from build123d import *

# Parameters (mm, degrees)
F1_DEPTH = 28
F3_DEPTH = 244
F5_DEPTH = 28
F6_R     = 2
F7_R     = 1
F8_R     = 4.25
F9_DEPTH = 25


with BuildPart() as f1:
    # F0 (on Top) → F1 (new body)
    with BuildSketch(Plane.XY):
        Polygon((-19.75, -17.750001), (-19.75, -19.75), (-9.25, -19.75), (19.75, 9.25), (19.75, 19.75), (17.750001, 19.75), (17.750001, 10.078427), (-10.078427, -17.750001), align=None)
    extrude(amount=F1_DEPTH)

    # F2 (on face) → F3 (join)
    with BuildSketch(Plane.XY.offset(28)):
        Polygon((-19.75, -19.75), (-9.25, -19.75), (19.75, 9.25), (19.75, 19.75), (11.25, 19.75), (11.25, 24.25), (9.25, 26.25), (9.25, 23.421573), (9.25, 19.75), (9.25, 17.750001), (17.750001, 17.750001), (17.750001, 10.078427), (16.585787, 8.914213), (-8.914213, -16.585787), (-10.078427, -17.750001), (-17.750001, -17.750001), (-17.750001, -9.25), (-19.75, -9.25), (-23.421573, -9.25), (-26.25, -9.25), (-24.25, -11.25), (-19.75, -11.25), align=None)
    extrude(amount=F3_DEPTH)

    # F4 (on face) → F5 (join)
    with BuildSketch(Plane.XY.offset(272)):
        Polygon((19.75, 9.25), (19.75, 19.75), (17.750001, 19.75), (17.750001, 10.078427), (-10.078427, -17.750001), (-19.75, -17.750001), (-19.75, -19.75), (-9.25, -19.75), align=None)
    extrude(amount=F5_DEPTH)

    # F6
    f6_edges = [f1.edges().sort_by_distance(p)[0] for p in [
        (19.75, 9.25, 150),
        (-9.25, -19.75, 150),
    ]]
    fillet(f6_edges, radius=F6_R)

    # F7
    f7_edges = [f1.edges().sort_by_distance(p)[0] for p in [
        (-19.75, -19.75, 150),
        (19.75, 19.75, 150),
    ]]
    fillet(f7_edges, radius=F7_R)

    # F8 (on face) → F9 (cut)
    with BuildSketch(Plane(origin=(5.25, -5.25, 0), x_dir=(0.707107, 0.707107, 0), z_dir=(0.707107, -0.707107, 0))):
        with Locations((0, 286)):
            Circle(F8_R)
    extrude(amount=-F9_DEPTH, mode=Mode.SUBTRACT)


solid = f1.part
Geometry check sheet. Reference: the model listing, model coordinates, mm. A direction names the side the tool comes from. Coordinates: 2 decimals unless noted, no trailing zeros. Order: outer loops, then holes, each group sorted by start corner. A loop starts at its lowest first (then second) coordinate and runs counter-clockwise, first axis right, second up. Notation, with made-up numbers: (-9.75, 39.5) - (45.25, 39.5) arc R17 cw to (45.25, 46.5) - close; hole circle Ø10 at (-22, 81). An arc over 180 degrees is marked (long way). Answer in a Markdown table with one row per item. Add a question column.
1) Gauge pin test, flat ends, axial feed: P1, Ø10.5, axis at y = 16, z = 159, coming from the -X side; P2, Ø1.3, axis at x = -22, z = 137.5, coming from the -Y side; P3, Ø7, axis at y = -14, z = 188.5, coming from the +X side; P4, Ø8, axis at x = 13.5, y = 10, coming from the +Z side. Record the tip position at first contact, or that the pin passes through.
2) Material ranges on line 1 along X through (y, z) = (18, 220); line 2 along Y through (x, z) = (13.5, 67); line 3 along Y through (x, z) = (16.5, 79), recorded low to high. Write a range as [from, to].
3) Set-up check for faces 4 (the flat face through (-19.75, -15, 148)), 5 (the flat face through (13, 17.75, 148)), 6 (the flat face through (9.25, 22, 148)), 7 (the flat face through (4.03, -3.64, 147.9)), 8 (the flat face through (12.2, 19.5, 28)): record each of +Z, -Z, +X, -X, +Y, -Y from which the full face is reachable in a straight line by a thin tool's end or side.
4) Release check for a two-part mould opening along Y. For faces 1 (the flat face through (15, 19.75, 148)), 2 (the flat face through (-19.5, -12.2, 28)), 3 (the flat face through (17.75, 14, 148)) record: +Y half, -Y half, draft (parallel to the pull), parting line (faces both ways), or undercut.
5) Cross-section at C-C, the plane x = -6. Record the cut outline in (y, z).
6) Cross-section at A-A, the plane z = 135. Record the cut outline in (x, y), then the cut area to 3 significant figures.
7) Cross-section at B-B, the plane z = 19. Record the cut outline in (x, y), then the cut area to 3 significant figures.
Check result:
| question | item | result |
|---|---|---|
| 1 | P1 | stops at x = 9.25 |
| 1 | P2 | stops at y = -11.25 |
| 1 | P3 | stops at x = 0 |
| 1 | P4 | stops at z = 300 |
| 2 | line 1 | x = [9.25, 19.75] |
| 2 | line 2 | y = [3, 5.83], [17.75, 19.75] |
| 2 | line 3 | y = [6, 8.83], [17.75, 19.75] |
| 3 | face 4 | +Z, -Z, -X, -Y |
| 3 | face 5 | +Z, -Z, -X |
| 3 | face 6 | +Z, -Z, -X, +Y |
| 3 | face 7 | +Z, -Z |
| 3 | face 8 | -Z, -X, +Y |
| 4 | face 1 | +Y half |
| 4 | face 2 | draft |
| 4 | face 3 | undercut |
| 5 | outline | (-16.5, 0) - (-13.67, 0) - (-13.67, 300) - (-16.5, 300) - close |
| 6 | outline | (-26.25, -9.25) - (-24.25, -11.25) - (-19.75, -11.25) - (-19.75, -18.75) arc R1 ccw to (-18.75, -19.75) - (-10.08, -19.75) arc R2 ccw to (-8.66, -19.16) - (19.16, 8.66) arc R2 ccw to (19.75, 10.08) - (19.75, 18.75) arc R1 ccw to (18.75, 19.75) - (11.25, 19.75) - (11.25, 24.25) - (9.25, 26.25) - (9.25, 17.75) - (17.75, 17.75) - (17.75, 10.08) - (-10.08, -17.75) - (-17.75, -17.75) - (-17.75, -9.25) - close |
| 6 | area | 176 mm² |
| 7 | outline | (-19.75, -18.75) arc R1 ccw to (-18.75, -19.75) - (-10.08, -19.75) arc R2 ccw to (-8.66, -19.16) - (19.16, 8.66) arc R2 ccw to (19.75, 10.08) - (19.75, 18.75) arc R1 ccw to (18.75, 19.75) - (17.75, 19.75) - (17.75, 10.08) - (-10.08, -17.75) - (-19.75, -17.75) - close |
| 7 | area | 120 mm² |
